```python
from build123d import *

# Parameters (mm, degrees)
SKETCH1_W           = 171.4
SKETCH1_H           = 57
BOSS_EXTRUDE1_DEPTH = 3
BOSS_EXTRUDE2_DEPTH = 30
SKETCH3_W           = 52
SKETCH3_H           = 25
CUT_EXTRUDE1_DEPTH  = 192
SKETCH4_W           = 171.4
SKETCH4_H           = 57
BOSS_EXTRUDE3_DEPTH = 3
SKETCH5_R           = 3.5
BOSS_EXTRUDE4_DEPTH = 8
SKETCH6_R           = 1.4
CUT_EXTRUDE2_DEPTH  = 6
SKETCH8_W           = 165.4
SKETCH8_H           = 25
CUT_EXTRUDE3_DEPTH  = 6
FILLET2_START       = -85.7
FILLET2_DEPTH       = 3
FILLET2_START_2     = 82.7
FILLET2_2_DEPTH     = 3
FILLET2_START_3     = -28.5
FILLET2_3_DEPTH     = 5
FILLET2_4_DEPTH     = 2
FILLET2_START_4     = -82.7
FILLET2_5_DEPTH     = 165.4
SKETCH9_W           = 55
SKETCH9_H           = 30
BOSS_EXTRUDE5_DEPTH = 19
SKETCH10_W          = 26
SKETCH10_H          = 17
CUT_EXTRUDE4_DEPTH  = 53


with BuildPart() as part:
    # Sketch1 → Boss-Extrude1 (new body)
    with BuildSketch(Plane(origin=(0, 0, 0), x_dir=(1, 0, 0), z_dir=(0, 1, 0))):
        Rectangle(SKETCH1_W, SKETCH1_H)
    extrude(amount=BOSS_EXTRUDE1_DEPTH)

    # Sketch2 → Boss-Extrude2 (add)
    with BuildSketch(Plane(origin=(0, 3, 0), x_dir=(1, 0, 0), z_dir=(0, 1, 0))):
        Polygon((-85.7, -28.5), (-82.7, -28.5), (-82.7, 26.5), (82.7, 26.5), (82.7, -28.5), (85.7, -28.5), (85.7, 28.5), (-85.7, 28.5), align=None)
    extrude(amount=BOSS_EXTRUDE2_DEPTH)

    # Sketch3 → Cut-Extrude1 (cut)
    with BuildSketch(Plane.ZY.offset(85.7)):
        with Locations((-0.5, 20.5)):
            Rectangle(SKETCH3_W, SKETCH3_H)
    extrude(amount=-CUT_EXTRUDE1_DEPTH, mode=Mode.SUBTRACT)

    # Sketch4 → Boss-Extrude3 (add)
    with BuildSketch(Plane(origin=(0, 33, 0), x_dir=(1, 0, 0), z_dir=(0, 1, 0))):
        Rectangle(SKETCH4_W, SKETCH4_H)
    extrude(amount=BOSS_EXTRUDE3_DEPTH)

    # Sketch5 → Boss-Extrude4 (add)
    with BuildSketch(Plane(origin=(0, 36, 0), x_dir=(1, 0, 0), z_dir=(0, 1, 0))):
        with Locations(Location((-60.7, 13.5, 0), (0, 0, 90))):
            Circle(SKETCH5_R)
        with Locations(Location((-40.7, 13.5, 0), (0, 0, 90))):
            Circle(SKETCH5_R)
        with Locations(Location((-40.7, -13.5, 0), (0, 0, 90))):
            Circle(SKETCH5_R)
        with Locations(Location((-60.7, -13.5, 0), (0, 0, 90))):
            Circle(SKETCH5_R)
        with Locations(Location((60.7, -13.5, 0), (0, 0, 90))):
            Circle(SKETCH5_R)
        with Locations(Location((40.7, -13.5, 0), (0, 0, 90))):
            Circle(SKETCH5_R)
        with Locations(Location((40.7, 13.5, 0), (0, 0, 90))):
            Circle(SKETCH5_R)
        with Locations(Location((60.7, 13.5, 0), (0, 0, 90))):
            Circle(SKETCH5_R)
    extrude(amount=BOSS_EXTRUDE4_DEPTH)

    # Sketch6 → Cut-Extrude2 (cut)
    with BuildSketch(Plane(origin=(0, 44, 0), x_dir=(1, 0, 0), z_dir=(0, 1, 0))):
        with Locations(Location((-60.7, 13.5, 0), (0, 0, 270))):
            Circle(SKETCH6_R)
        with Locations(Location((-40.7, 13.5, 0), (0, 0, 270))):
            Circle(SKETCH6_R)
        with Locations(Location((-40.7, -13.5, 0), (0, 0, 90))):
            Circle(SKETCH6_R)
        with Locations(Location((-60.7, -13.5, 0), (0, 0, 90))):
            Circle(SKETCH6_R)
        with Locations(Location((60.7, -13.5, 0), (0, 0, 270))):
            Circle(SKETCH6_R)
        with Locations(Location((40.7, -13.5, 0), (0, 0, 270))):
            Circle(SKETCH6_R)
        with Locations(Location((40.7, 13.5, 0), (0, 0, 90))):
            Circle(SKETCH6_R)
        with Locations(Location((60.7, 13.5, 0), (0, 0, 90))):
            Circle(SKETCH6_R)
    extrude(amount=-CUT_EXTRUDE2_DEPTH, mode=Mode.SUBTRACT)

    # Sketch8 → Cut-Extrude3 (cut)
    with BuildSketch(Plane(origin=(0, 0, -28.5), x_dir=(-1, 0, 0), z_dir=(0, 0, -1))):
        with Locations((0, 20.5)):
            Rectangle(SKETCH8_W, SKETCH8_H)
    extrude(amount=-CUT_EXTRUDE3_DEPTH, mode=Mode.SUBTRACT)

    # Fillet2: read off the stored shape, not the designer's step
    # Fillet2 outline → Fillet2 (add)
    with BuildSketch(Plane.YZ.offset(FILLET2_START)):
        with BuildLine():
            ThreePointArc((33, -23.5), (32.121320344, -25.621320344), (30, -26.5))
            Line((30, -26.5), (33, -26.5))
            Line((33, -26.5), (33, -23.5))
        make_face()
        with BuildLine():
            ThreePointArc((30, 25.5), (32.121320344, 24.621320344), (33, 22.5))
            Line((33, 22.5), (33, 25.5))
            Line((33, 25.5), (30, 25.5))
        make_face()
        with BuildLine():
            Line((8, 25.5), (8, 22.5))
            ThreePointArc((8, 22.5), (8.878679656, 24.621320344), (11, 25.5))
            Line((11, 25.5), (8, 25.5))
        make_face()
    extrude(amount=FILLET2_DEPTH)

    # Fillet2 2 outline → Fillet2 2 (add)
    with BuildSketch(Plane.YZ.offset(FILLET2_START_2)):
        with BuildLine():
            ThreePointArc((33, -23.5), (32.121320344, -25.621320344), (30, -26.5))
            Line((30, -26.5), (33, -26.5))
            Line((33, -26.5), (33, -23.5))
        make_face()
        with BuildLine():
            ThreePointArc((30, 25.5), (32.121320344, 24.621320344), (33, 22.5))
            Line((33, 22.5), (33, 25.5))
            Line((33, 25.5), (30, 25.5))
        make_face()
        with BuildLine():
            Line((8, 25.5), (8, 22.5))
            ThreePointArc((8, 22.5), (8.878679656, 24.621320344), (11, 25.5))
            Line((11, 25.5), (8, 25.5))
        make_face()
    extrude(amount=FILLET2_2_DEPTH)

    # Fillet2 3 outline → Fillet2 3 (add)
    with BuildSketch(Plane.XY.offset(FILLET2_START_3)):
        with BuildLine():
            Line((82.7, 33), (79.7, 33))
            ThreePointArc((79.7, 33), (81.821320344, 32.121320344), (82.7, 30))
            Line((82.7, 30), (82.7, 33))
        make_face()
        with BuildLine():
            ThreePointArc((-82.7, 30), (-81.821320344, 32.121320344), (-79.7, 33))
            Line((-79.7, 33), (-82.7, 33))
            Line((-82.7, 33), (-82.7, 30))
        make_face()
    extrude(amount=FILLET2_3_DEPTH)

    # Fillet2 4 outline → Fillet2 4 (add)
    with BuildSketch(Plane.XY.offset(FILLET2_START_3)):
        with BuildLine():
            Line((82.7, 8), (82.7, 11))
            ThreePointArc((82.7, 11), (81.821320344, 8.878679656), (79.7, 8))
            Line((79.7, 8), (82.7, 8))
        make_face()
        with BuildLine():
            ThreePointArc((-79.7, 8), (-81.821320344, 8.878679656), (-82.7, 11))
            Line((-82.7, 11), (-82.7, 8))
            Line((-82.7, 8), (-79.7, 8))
        make_face()
    extrude(amount=FILLET2_4_DEPTH)

    # Fillet2 5 outline → Fillet2 5 (cut)
    with BuildSketch(Plane.YZ.offset(FILLET2_START_4)):
        with BuildLine():
            Line((30, -23.5), (30, -26.5))
            ThreePointArc((30, -26.5), (32.121320344, -25.621320344), (33, -23.5))
            Line((33, -23.5), (30, -23.5))
        make_face()
    extrude(amount=FILLET2_5_DEPTH, mode=Mode.SUBTRACT)

    # Sketch9 → Boss-Extrude5 (add)
    with BuildSketch(Plane.XZ):
        with Locations((-58.2, 0)):
            Rectangle(SKETCH9_W, SKETCH9_H)
    extrude(amount=BOSS_EXTRUDE5_DEPTH)

    # Sketch10 → Cut-Extrude4 (cut)
    with BuildSketch(Plane.ZY.offset(85.7)):
        with Locations((0, -8.5)):
            Rectangle(SKETCH10_W, SKETCH10_H)
    extrude(amount=-CUT_EXTRUDE4_DEPTH, mode=Mode.SUBTRACT)


solid = part.part
```
Here's how the part is built. I have some questions about the finished solid (model axes, mm). A direction names the side the tool comes from. Round coordinates to 2 decimals unless told otherwise and drop trailing zeros. Loops run counter-clockwise (first coordinate to the right, second up) from the corner with the lowest first, then second, coordinate; pieces in that order, holes last. Notation, with made-up numbers: (17.5, 36.5) -> (76.5, 36.5) arc R20 ccw to (76.5, 70.5) -> close; hole circle Ø6 at (-0.5, 55.25). An arc over 180 degrees is marked (long way). Answer as CSV lines item,"result". Start each with the question number.
1. I'm going to push flat-ended pins straight in: P1, Ø2, axis at x = -29, y = 10, coming from the +Z side; P2, Ø2.5, axis at x = 84, z = -0.5, coming from the +Y side; P3, Ø21, axis at y = -11.5, z = 0.5, coming from the +X side; P4, Ø1.5, axis at x = -2, z = -8.5, coming from the -Y side. Where does each tip first touch, or does it pass through?
2. Imagine slicing it at B-B on x = -1.5. Write out the boundary of the cut face in (y, z), plus the area to 3 significant figures.
3. For faces 1 (the face through (83.32, 32.48, -25.19)), 2 (the face through (43.805, 39.944, 11.885)), 3 (the face through (-59, -9, -15)), which set-ups out of +Z, -Z, +X, -X, +Y, -Y let a thin tool reach every point of the face, with its end or its side?
4. If we mould it in two halves opening along Y, with no side actions, what happens to faces 4 (the face through (-81.448, 32.438, -26.591)), 5 (the face through (-13, 34, 28.5)), 6 (the face through (-39, 44, 14))? For each: pulls with the +Y half, pulls with the -Y half, needs draft (parallel to the pull), parting line crosses it, or undercut.
5. Imagine slicing it at A-A on z = -5.5. Write out the boundary of the cut face in (x, y).
6. Imagine slicing it at C-C on y = 16.5. Write out the boundary of the cut face in (x, z).
7. I need wall thicknesses on probe 1 along Y at (x, z) = (-20, 15); probe 2 along Z at (x, y) = (-60, 39); probe 3 along X at (y, z) = (4.5, 23). Which ranges of each line are inside material? Lowest first, please. Write a range as from..to.
Solution:
1,P1,"through"
1,P2,"y = 36"
1,P3,"x = -30.7"
1,P4,"y = 0"
2,outline,"(0, -28.5) -> (8, -28.5) -> (8, -26.5) -> (3, -26.5) -> (3, 28.5) -> (0, 28.5) -> close; (33, -28.5) -> (36, -28.5) -> (36, 28.5) -> (33, 28.5) -> close"
2,area,"352 mm²"
3,face 1,"+X, -X"
3,face 2,"+Y"
3,face 3,"-Z, +X, -X, -Y"
4,face 4,"undercut"
4,face 5,"needs draft"
4,face 6,"pulls with the +Y half"
5,outline,"(-85.7, -19) -> (-30.7, -19) -> (-30.7, 0) -> (85.7, 0) -> (85.7, 8) -> (82.7, 8) -> (82.7, 3) -> (-82.7, 3) -> (-82.7, 8) -> (-85.7, 8) -> (-85.7, 0) -> (-32.7, 0) -> (-32.7, -17) -> (-85.7, -17) -> close; (-85.7, 33) -> (85.7, 33) -> (85.7, 36) -> (-85.7, 36) -> close"
6,outline,"(-85.7, -28.5) -> (-82.7, -28.5) -> (-82.7, -26.5) -> (-85.7, -26.5) -> close; (-85.7, 25.5) -> (-82.7, 25.5) -> (-82.7, 28.5) -> (-85.7, 28.5) -> close; (82.7, -28.5) -> (85.7, -28.5) -> (85.7, -26.5) -> (82.7, -26.5) -> close; (82.7, 25.5) -> (85.7, 25.5) -> (85.7, 28.5) -> (82.7, 28.5) -> close"
7,probe 1,"0..3, 33..36"
7,probe 2,"-16.93..-14.71, -12.29..-10.07, 10.07..12.29, 14.71..16.93"
7,probe 3,"-85.7..-82.7, 82.7..85.7"
